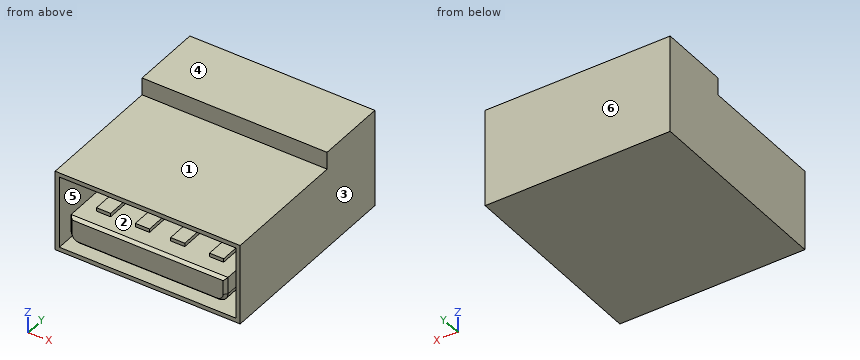
Autodesk Inventor part; units mm, degrees
ref_plane "YZ Plane" through (0, 0, 0) normal (1, 0, 0) x (0, 1, 0)
ref_plane "XZ Plane" through (0, 0, 0) normal (0, 1, 0) x (-1, 0, 0)
ref_plane "XY Plane" through (0, 0, 0) normal (0, 0, 1) x (1, 0, 0)
sketch "Sketch1" plane through (0, 0, 0) normal (0, 0, 1) x (1, 0, 0)
  line L0 (-6.55, 7.05) -> (6.55, 7.05)
  line L1 (6.55, 7.05) -> (6.55, -7.05)
  line L2 (6.55, -7.05) -> (-6.55, -7.05)
  line L3 (-6.55, -7.05) -> (-6.55, 7.05)
  point P0 (0, 0)
  point P1 (-6.55, 0)
  point P2 (0, 7.05)
  dimension "d0" = 13.1
  dimension "d1" = 14.1
extrude "Extrusion1" add sketch "Sketch1" along normal blind 5.72
sketch "Sketch2" plane through (0, 0, 5.72) normal (0, 0, 1) x (1, 0, 0)
  line L0 (6.55, 7.05) -> (6.55, -7.05)
  line L1 (-6.55, 7.05) -> (6.55, 7.05)
  line L2 (6.55, 7.05) -> (6.55, 2.05)
  line L3 (6.55, 2.05) -> (-6.55, 2.05)
  line L4 (-6.55, 2.05) -> (-6.55, 7.05)
  point P0 (0, 0)
  dimension "d4" = 5
extrude "Extrusion2" add sketch "Sketch2" along normal blind 1.23
sketch "Sketch3" plane through (-6.55, -7.05, 0) normal (0, -1, 0) x (1, 0, 0)
  line L0 (13.1, 5.72) -> (0, 5.72)
  line L1 (0, 0) -> (0, 5.72)
  line L2 (13.1, 0) -> (0, 0)
  line L3 (13.1, 0) -> (13.1, 5.72)
  line L4 (0.3, 5.42) -> (12.8, 5.42)
  line L5 (12.8, 5.42) -> (12.8, 0.3)
  line L6 (12.8, 0.3) -> (0.3, 0.3)
  line L7 (0.3, 0.3) -> (0.3, 5.42)
  line L8 (1, 2.86) -> (12.1, 2.86)
  line L9 (12.1, 2.86) -> (12.1, 1.02)
  line L10 (12.1, 1.02) -> (1, 1.02)
  line L11 (1, 1.02) -> (1, 2.86)
  line L12 (2.05, 2.86) -> (3.05, 2.86)
  line L13 (4.8, 2.86) -> (5.8, 2.86)
  line L14 (7.3, 2.86) -> (8.3, 2.86)
  line L15 (10.05, 2.86) -> (11.05, 2.86)
  point P0 (6.55, 0)
  dimension "d7" = 0.3
  dimension "d9" = 5.72
  dimension "d10" = 5.12
  dimension "d11" = 0.7
  dimension "d13" = 1.84
  dimension "d14" = 0.7
  dimension "d17" = 2.56
extrude "Extrusion3" cut sketch "Sketch3" against normal blind 10.3 contours L4 L5 L6 L7
fillet "Fillet3" radius 0.64 1 edges at (5.55, -1.9, 1.02)
fillet "Fillet4" radius 0.64 1 edges at (-5.55, -1.9, 1.02)
chamfer "Chamfer1" distance 0.2 angle 45 5 edges at (5.55, -7.05, 2.26) (5.3625, -7.05, 1.2075) (0, -7.05, 1.02) (-5.3625, -7.05, 1.2075) (-5.55, -7.05, 2.26)
chamfer "Chamfer7" distance 0.2 angle 45 1 edges at (0, -7.05, 2.86)
sketch "Sketch4" plane through (-6.55, 3.25, 0) normal (0, -1, 0) x (1, 0, 0)
  line L0 (12.1, 2.86) -> (1, 2.86)
  line L1 (12.1, 1.66) -> (12.1, 2.86)
  line L2 (2.05, 2.86) -> (3.05, 2.86)
  line L3 (3.05, 2.86) -> (3.05, 3.11)
  line L4 (3.05, 3.11) -> (2.05, 3.11)
  line L5 (2.05, 3.11) -> (2.05, 2.86)
  line L6 (4.8, 2.86) -> (5.8, 2.86)
  line L7 (5.8, 2.86) -> (5.8, 3.11)
  line L8 (5.8, 3.11) -> (4.8, 3.11)
  line L9 (4.8, 3.11) -> (4.8, 2.86)
  line L10 (7.3, 2.86) -> (8.3, 2.86)
  line L11 (8.3, 2.86) -> (8.3, 3.11)
  line L12 (8.3, 3.11) -> (7.3, 3.11)
  line L13 (7.3, 3.11) -> (7.3, 2.86)
  line L14 (10.05, 2.86) -> (11.05, 2.86)
  line L15 (11.05, 2.86) -> (11.05, 3.11)
  line L16 (11.05, 3.11) -> (10.05, 3.11)
  line L17 (10.05, 3.11) -> (10.05, 2.86)
  point P0 (6.55, 0)
  dimension "d57" = 1
  dimension "d58" = 1
  dimension "d59" = 1
  dimension "d60" = 1
  dimension "d61" = 0.25
  dimension "d62" = 0.25
  dimension "d63" = 0.25
  dimension "d64" = 0.25
  dimension "d65" = 1.5
  dimension "d66" = 1.75
  dimension "d67" = 1.75
  dimension "d68" = 1.05
extrude "Extrusion5" add sketch "Sketch4" along normal blind 9
properties part number "usb host con"
The listing builds one solid part. Answer for the finished solid, in the listing's coordinates (mm). Face numbers are marked on the shaded views. A direction names the side the tool comes from. Give positions to 0.01 mm unless a question says otherwise; leave off trailing zeros. Loops run counter-clockwise (first coordinate to the right, second up) from the corner with the lowest first, then second, coordinate; pieces in that order, holes last. Notation, with made-up numbers: M 42,0 L 82,0 A13 ccw 82,6 Z; hole C 88.5,60 d7. An arc over 180 degrees is marked long. One line per item, written item: value.
Q1. A cutting plane is placed at A-A on y = -6. Determine the outline of the cut face in (x, z), then the cut area to 3 significant figures.
Working result:
outline: M -6.55,0 L 6.55,0 L 6.55,5.72 L -6.55,5.72 Z; M -5.55,1.66 A0.64 ccw -4.91,1.02 L 4.91,1.02 A0.64 ccw 5.55,1.66 L 5.55,2.86 L -5.55,2.86 Z; hole M -6.25,0.3 L 6.25,0.3 L 6.25,5.42 L -6.25,5.42 Z
area: 31.2 mm^2
Q2. A cutting plane is placed at B-B on z = 4. Determine the outline of the cut face in (x, y), then the cut area to 3 significant figures.
Working result:
outline: M -6.55,-7.05 L -6.25,-7.05 L -6.25,3.25 L 6.25,3.25 L 6.25,-7.05 L 6.55,-7.05 L 6.55,7.05 L -6.55,7.05 Z
area: 56.0 mm^2
Q3. For the marked faces 1, 2 and 3, determine the directions among +Z, -Z, +X, -X, +Y, -Y from which every point of the face is accessible in a straight line to the end or side of a thin tool.
Working result:
face 1: +Z, +X, -X, -Y
face 2: -Y
face 3: +Z, -Z, +X, +Y, -Y
Q4. A cutting plane is placed at D-D on y = -0.5. Give the number of separate pieces and of enclosed holes in the cut face, then the cut area to 3 significant figures.
Working result:
separate pieces: 2
enclosed holes: 1
area: 32.2 mm^2
Q5. Determine the mould class of the marked faces 4, 5 and 6 for opening direction Z: +Z half, -Z half, draft (parallel to the pull), parting line (faces both ways), or undercut.
Working result:
face 4: +Z half
face 5: undercut
face 6: draft
Q6. Find the intervals of material crossed by line 1 (Z direction, x = 3, y = 2); line 2 (X direction, y = -0.5, z = 2.5); line 3 (Z direction, x = 1.5, y = -2.25), in increasing order. Write a range as from..to.
Working result:
line 1: z = 0..0.3, 1.02..2.86, 5.42..5.72
line 2: x = -6.55..-6.25, -5.55..5.55, 6.25..6.55
line 3: z = 0..0.3, 1.02..3.11, 5.42..5.72
Q7. A cutting plane is placed at C-C on x = 3.25. Determine the outline of the cut face in (y, z), then the cut area to 3 significant figures.
Working result:
outline: M -7.05,0 L 7.05,0 L 7.05,6.95 L 2.05,6.95 L 2.05,5.72 L -7.05,5.72 L -7.05,5.42 L 3.25,5.42 L 3.25,2.86 L -6.85,2.86 L -7.05,2.66 L -7.05,1.22 L -6.85,1.02 L 3.25,1.02 L 3.25,0.3 L -7.05,0.3 Z
area: 53.0 mm^2
Q8. A flat-ended cylindrical pin translates along its axis: P1, Ø4.5, axis at x = -1, y = -0.5, coming from the +Z side. Find the tip coordinate at first contact, or state that the pin passes through.
Working result:
P1: stops at z = 5.72
